Autodesk Inventor part; units mm, degrees
ref_plane "YZ Plane" through (0, 0, 0) normal (1, 0, 0) x (0, 1, 0)
ref_plane "XZ Plane" through (0, 0, 0) normal (0, 1, 0) x (-1, 0, 0)
ref_plane "XY Plane" through (0, 0, 0) normal (0, 0, 1) x (1, 0, 0)
sketch "Sketch1" plane through (0, 0, 0) normal (1, 0, 0) x (0, 1, 0)
  line L0 (0, 0) -> (0, 300)
  circle A0 centre (0, 300) radius 25
  circle A1 centre (0, 0) radius 25
  circle A2 centre (0, 300) radius 10
  circle A3 centre (0, 0) radius 10
  line L1 (25, 300) -> (25, 0)
  line L2 (-25, 0) -> (-25, 300)
  dimension "d0" = 300
  dimension "d1" = 50
  dimension "d2" = 20
extrude "Extrusion1" add sketch "Sketch1" along normal blind 70 contours A1 | A1 L2 A0 L0 | L0 A0 L1 A1 | A2 | A0
sketch "Sketch2" plane through (0, 25, 300) normal (0, 1, 0) x (1, 0, 0)
  line L0 (0, -25) -> (0, 0)
  line L1 (70, 300) -> (70, 325)
  line L2 (0, 0) -> (70, 0)
  line L3 (70, 0) -> (70, 300)
  line L4 (70, 300) -> (0, 300)
  line L5 (0, 300) -> (0, 0)
  line L6 (10, 10) -> (60, 10)
  line L7 (60, 10) -> (60, 290)
  line L8 (60, 290) -> (10, 290)
  line L9 (10, 290) -> (10, 10)
  line L10 (0, 325) -> (70, 325)
  line L11 (10, 290) -> (60, 290)
  line L12 (60, 290) -> (60, 325)
  line L13 (60, 325) -> (10, 325)
  line L14 (10, 325) -> (10, 290)
  line L15 (0, -25) -> (70, -25)
  line L16 (10, 10) -> (60, 10)
  line L17 (60, 10) -> (60, -25)
  line L18 (60, -25) -> (10, -25)
  line L19 (10, -25) -> (10, 10)
  line L20 (60, 260) -> (10, 260)
  line L21 (10, 260) -> (10, 40)
  line L22 (10, 40) -> (60, 40)
  line L23 (60, 40) -> (60, 260)
  line L24 (60, 325) -> (10, 325)
  line L25 (10, 325) -> (10, 270)
  line L26 (10, 270) -> (60, 270)
  line L27 (60, 270) -> (60, 325)
  line L28 (60, -25) -> (10, -25)
  line L29 (10, -25) -> (10, 30)
  line L30 (10, 30) -> (60, 30)
  line L31 (60, 30) -> (60, -25)
  point P0 (60, 40)
  point P1 (10, 260)
  point P2 (60, 270)
  dimension "d5" = 10
  dimension "d6" = 10
  dimension "d9" = 30
  dimension "d10" = 30
  dimension "d13" = 10
  dimension "d14" = 10
extrude "Extrusion2" cut sketch "Sketch2" against normal through all contours L14 L10 L12 L4 | L4 L12 L8 L14 | L8 L7 L26 L9
extrude "Extrusion3" cut sketch "Sketch2" against normal through all contours L9 L20 L7 L22
properties part number "arm2"
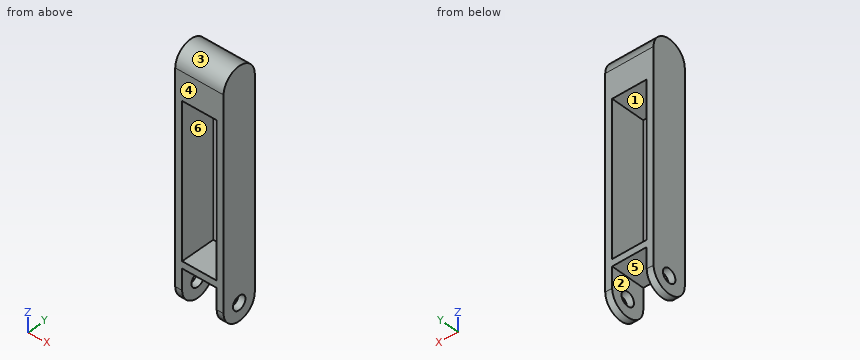
For this review, take the finished solid that the model builds, in its own axes (mm). Face numbers are marked on the shaded views. A direction names the side the tool comes from. Coordinates: 2 decimals unless noted, no trailing zeros. Order: outer loops, then holes, each group sorted by start corner. A loop starts at its lowest first (then second) coordinate and runs counter-clockwise, first axis right, second up. Notation, with made-up numbers: (38, 26.25) - (67, 26.25) arc R20 cw to (67, 31.25) - close; hole circle Ø7 at (77.5, -16). An arc over 180 degrees is marked (long way). Answer as CSV lines item,"result". Start each with the question number.
1) Add section D-D (y = -16.5). State the section outline as (x, z) points.
2) To check wall thickness, follow line 1 along X through (y, z) = (-9, 52); line 2 along Y through (x, z) = (67, 0); line 3 along Z through (x, y) = (63, 0). State the ranges of each line that lie inside material, in increasing order. Write a range as [from, to].
3) Insertion check: P1, Ø25, axis at y = -10, z = 5.5, coming from the -X side; P2, Ø8, axis at x = 50, y = -1, coming from the +Z side; P3, Ø3, axis at x = 48, y = -16, coming from the +Z side; P4, Ø3, axis at x = 35, y = 6.5, coming from the -Z side. Each pin has a flat end and moves straight along its axis. Give the tip position at first contact, or say it passes through.
4) Add section C-C (z = 93). State the section outline as (x, y) points, then the cut area to 3 significant figures.
5) Machinability: for the marked faces 1, 2 and 3, which of the approach directions +Z, -Z, +X, -X, +Y, -Y give a long, thin tool a straight path to every point of the face, cutting with its end or side? Answer none if there is none.
6) Add section B-B (x = 28.5). State the section outline as (y, z) points.
7) Add section A-A (y = 0). State the section outline as (x, z) points.
8) Draft analysis for pull direction Z (two halves, no side actions). For the marked faces 4, 5 and 6, state which applies: +Z half, -Z half, draft (parallel to the pull), parting line (faces both ways), or undercut.
Result:
1,outline,"(0, -18.78) - (10, -18.78) - (10, 30) - (60, 30) - (60, -18.78) - (70, -18.78) - (70, 318.78) - (0, 318.78) - close; hole (10, 40) - (60, 40) - (60, 260) - (10, 260) - close"
2,line 1,"[0, 10], [60, 70]"
2,line 2,"[-25, -10], [10, 25]"
2,line 3,"[-25, -10], [10, 325]"
3,P1,"x = 0"
3,P2,"z = 325"
3,P3,"z = 320.37"
3,P4,"z = 30"
4,outline,"(0, -25) - (10, -25) - (10, 25) - (0, 25) - close; (60, -25) - (70, -25) - (70, 25) - (60, 25) - close"
4,area,"1,000 mm^2"
5,face 1,"+Y, -Y"
5,face 2,"-Z, +Y, -Y"
5,face 3,"+Z, +X, -X"
6,outline,"(-25, 30) - (25, 30) - (25, 40) - (-25, 40) - close; (-25, 260) - (25, 260) - (25, 300) arc R25 ccw to (-25, 300) - close"
7,outline,"(0, -25) - (10, -25) - (10, -10) - (0, -10) - close; (0, 10) - (10, 10) - (10, 30) - (60, 30) - (60, 10) - (70, 10) - (70, 325) - (0, 325) - close; (60, -25) - (70, -25) - (70, -10) - (60, -10) - close; hole (10, 40) - (60, 40) - (60, 260) - (10, 260) - close"
8,face 4,"draft"
8,face 5,"-Z half"
8,face 6,"undercut"
